Design review of the part shown in the three views and the two pictorial views. Dimensions are in mm from the part's minimum x, y and z. Give positions to 0.01 mm unless a question says otherwise; leave off trailing zeros. Loops run counter-clockwise (first coordinate to the right, second up) from the corner with the lowest first, then second, coordinate; pieces in that order, holes last. Notation, with made-up numbers: (63, -30.75) -> (76, -30.75) arc R25 ccw to (76, -6.75) -> close; hole circle Ø4 at (58, 14). An arc over 180 degrees is marked (long way). Use CSV: the item, a comma, the result in double quotes. Start each with the question number.
Item 1: The part is to be moulded in two halves that separate along X. For the marked faces 1, 2 and 3, say which applies: +X half, -X half, draft (parallel to the pull), parting line (faces both ways), or undercut.
Item 2: We need section B-B (y = 12.94). State the section outline as (x, z) points, plus the area to 3 significant figures.
Item 3: We need section A-A (x = 12.6). State the section outline as (y, z) points, plus the area to 3 significant figures.
Item 4: We need section C-C (z = 2.2). State the section outline as (x, y) points, plus the area to 3 significant figures.
Item 5: Wall thickness on line 1 along Y through (x, z) = (12.6, 2.2); line 2 along Y through (x, z) = (9, 2.1); line 3 along X through (y, z) = (10.5, 2.25): over which ranges is each line inside the solid? List them lowest first. Write a range as from..to.
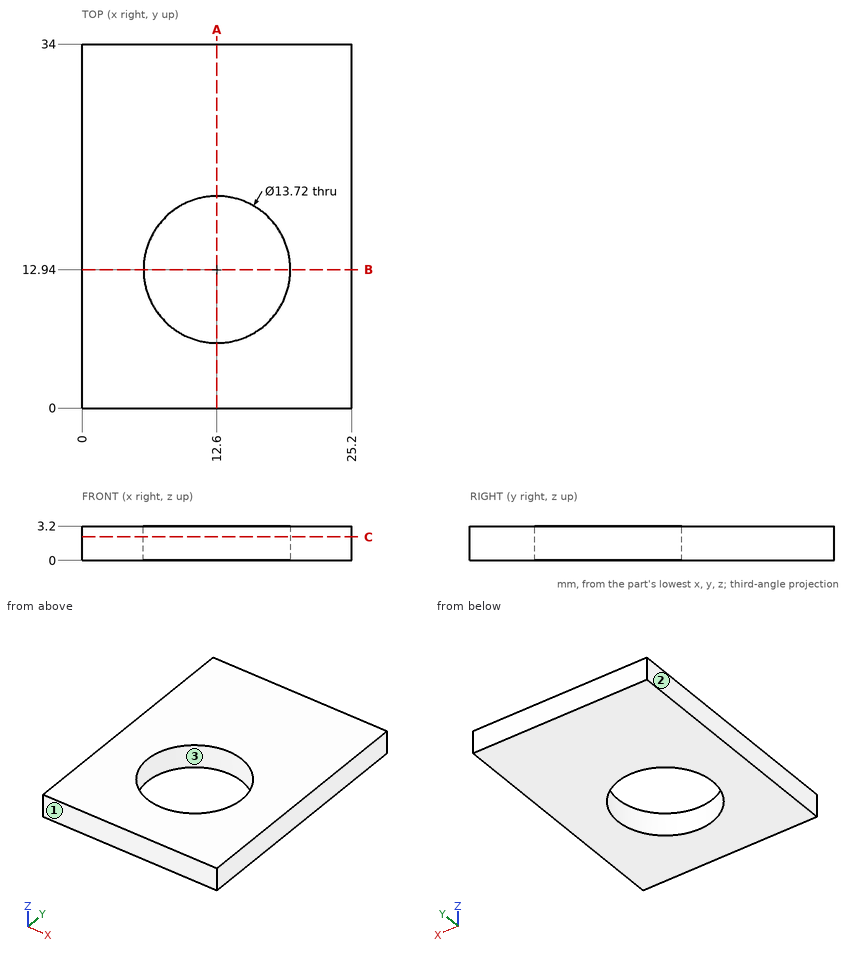
Results found:
1,face 1,"draft"
1,face 2,"-X half"
1,face 3,"undercut"
2,outline,"(0, 0) -> (5.74, 0) -> (5.74, 3.2) -> (0, 3.2) -> close; (19.46, 0) -> (25.2, 0) -> (25.2, 3.2) -> (19.46, 3.2) -> close"
2,area,"36.7 mm²"
3,outline,"(0, 0) -> (6.08, 0) -> (6.08, 3.2) -> (0, 3.2) -> close; (19.8, 0) -> (34, 0) -> (34, 3.2) -> (19.8, 3.2) -> close"
3,area,"64.9 mm²"
4,outline,"(0, 0) -> (25.2, 0) -> (25.2, 34) -> (0, 34) -> close; hole circle Ø13.72 at (12.6, 12.94)"
4,area,"709 mm²"
5,line 1,"0..6.08, 19.8..34"
5,line 2,"0..7.1, 18.78..34"
5,line 3,"0..6.19, 19.01..25.2"
